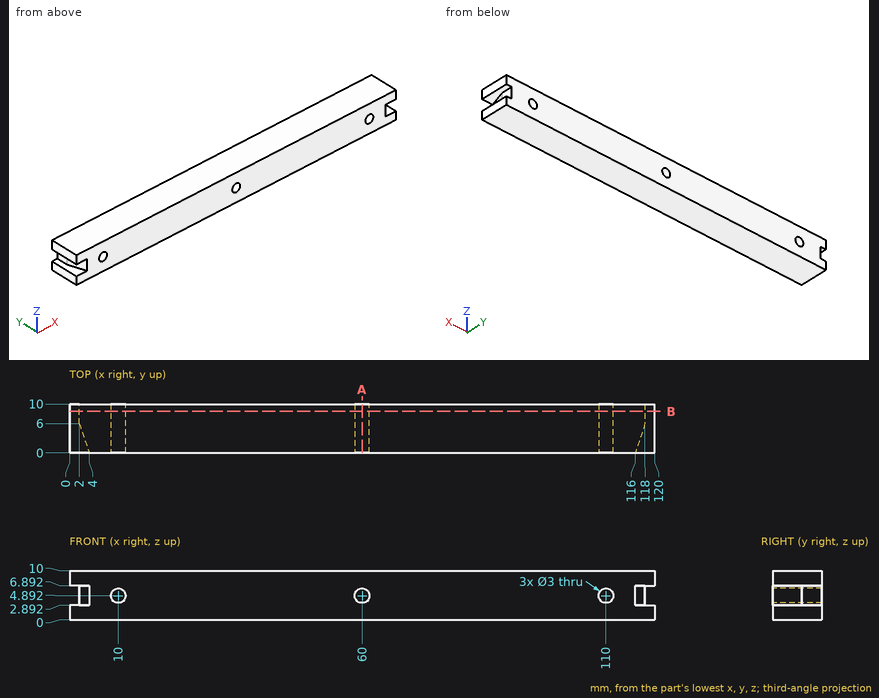
Drawing for the job (mm, zero at the part's lowest x, y, z). Give positions to 0.01 mm unless a question says otherwise; leave off trailing zeros. Order: outer loops, then holes, each group sorted by start corner. A loop starts at its lowest first (then second) coordinate and runs counter-clockwise, first axis right, second up. Notation, with made-up numbers: M -5,54.25 L 21,54.25 A15 cw 21,70.25 Z; hole C 42.5,45 d6. An arc over 180 degrees is marked long. Write item = value, one per line. Start each with the question number.
(1) Probe L1, parallel to X at y = 8, z = 4.75; L2, parallel to Z at x = 110, y = 5.25; L3, parallel to X at y = 9, z = 4. List the from-to ranges inside material, lowest first. Write a range as [from, to].
(2) Pin check, flat tips, straight feed: pin 1 Ø3 at (y, z) = (8, 5) entering from -X; pin 2 Ø1.8 at (x, z) = (10, 4.89) entering from -Y. Stop position of each tip, or through.
(3) Slice it at A-A on x = 60. Write the cut outline in (y, z), plus the area to 3 significant figures.
(4) Slice it at B-B on y = 8.5. Write the cut outline in (x, z), plus the area to 3 significant figures.
Responses:
q1.L1 = [2, 8.51], [11.49, 58.51], [61.49, 108.51], [111.49, 118]
q1.L2 = [0, 3.39], [6.39, 10]
q1.L3 = [2, 8.79], [11.21, 58.79], [61.21, 108.79], [111.21, 118]
q2.pin_1 = 2
q2.pin_2 = through
q3.outline = M 0,0 L 10,0 L 10,3.39 L 0,3.39 Z; M 0,6.39 L 10,6.39 L 10,10 L 0,10 Z
q3.area = 70.0 mm2
q4.outline = M 0,0 L 120,0 L 120,2.89 L 118,2.89 L 118,6.89 L 120,6.89 L 120,10 L 0,10 L 0,6.89 L 2,6.89 L 2,2.89 L 0,2.89 Z; hole C 10,4.89 d3; hole C 60,4.89 d3; hole C 110,4.89 d3
q4.area = 1,160 mm2
